from build123d import *

# Parameters (mm, degrees)
BOARDBASE_DEPTH      = 1.6
SKETCH2_R            = 1.75
SKETCH2_R_2          = 2.25
EXISTING_HOLES_DEPTH = 2.6
SKETCH3_W            = 30
SKETCH3_H            = 21
FREE_AREA_DEPTH      = 0.6


with BuildPart() as part:
    # Sketch1 → BoardBase (new body)
    with BuildSketch(Plane.XY):
        Polygon((9, 0), (99, 0), (99, 90), (0, 90), (0, 33), (9, 33), align=None)
    extrude(amount=-BOARDBASE_DEPTH)

    # Sketch2 → Existing Holes (cut, through all)
    with BuildSketch(Plane.XY):
        with Locations((9, 83)):
            Circle(SKETCH2_R)
        with Locations((43, 80.5)):
            Circle(SKETCH2_R_2)
        with Locations((43, 33)):
            Circle(SKETCH2_R_2)
    extrude(amount=-EXISTING_HOLES_DEPTH, mode=Mode.SUBTRACT)

    # Sketch3 → 'Free' area (add)
    with BuildSketch(Plane.XY):
        with Locations((84, 52.5)):
            Rectangle(SKETCH3_W, SKETCH3_H)
    extrude(amount=FREE_AREA_DEPTH)


solid = part.part
Model file for the job. Use its own axes, mm. Round coordinates to 2 decimals unless told otherwise and drop trailing zeros. Order: outer loops, then holes, each group sorted by start corner. A loop starts at its lowest first (then second) coordinate and runs counter-clockwise, first axis right, second up.
(1) Pin check, flat tips, straight feed: pin 1 (0.8 mm diameter, centred on y = 18, z = -1, fed in from -X); pin 2 (0.7 mm diameter, centred on x = 79, z = 0, fed in from -Y); pin 3 (0.5 mm diameter, centred on x = 79, z = 0.5, fed in from +Y); pin 4 (0.7 mm diameter, centred on y = 55.5, z = 0.5, fed in from -X). Stop position of each tip, or through.
(2) Band-saw the part on D-D (x = 83). List the corners of the cut face in (y, z), then the cut area to 3 significant figures.
(3) Band-saw the part on B-B (z = -1.1). List the corners of the cut face in (x, y).
(4) Band-saw the part on C-C (y = 67). List the corners of the cut face in (x, z).
(5) Pull direction Y, two halves, no side cores. Call faces 1 (the face through (49, 46, -1.6)), 2 (the face through (8.62, 81.29, -0.79)): released by +Y, released by -Y, zero draft, split by the parting line, or undercut.
(6) Band-saw the part on A-A (x = 43). List the corners of the cut face in (y, z).
(7) Drill centre lines: line 1 (Y direction, x = 43, z = -0.9); line 2 (Z direction, x = 16.5, y = 84.5); line 3 (Y direction, x = 45, z = -1.35). Where is each one in solid material? Low to high.
Verdict:
1. pin 1: stops at x = 9
1. pin 2: stops at y = 0
1. pin 3: stops at y = 63
1. pin 4: stops at x = 69
2. outline: (0, -1.6) - (90, -1.6) - (90, 0) - (63, 0) - (63, 0.6) - (42, 0.6) - (42, 0) - (0, 0) - close
2. area: 157 mm2
3. outline: (0, 33) - (9, 33) - (9, 0) - (99, 0) - (99, 90) - (0, 90) - close; hole circle Ø3.5 at (9, 83); hole circle Ø4.5 at (43, 33); hole circle Ø4.5 at (43, 80.5)
4. outline: (0, -1.6) - (99, -1.6) - (99, 0) - (0, 0) - close
5. face 1: zero draft
5. face 2: undercut
6. outline: (0, -1.6) - (30.75, -1.6) - (30.75, 0) - (0, 0) - close; (35.25, -1.6) - (78.25, -1.6) - (78.25, 0) - (35.25, 0) - close; (82.75, -1.6) - (90, -1.6) - (90, 0) - (82.75, 0) - close
7. line 1: y = 0 to 30.75, 35.25 to 78.25, 82.75 to 90
7. line 2: z = -1.6 to 0
7. line 3: y = 0 to 31.97, 34.03 to 79.47, 81.53 to 90
